```python
from build123d import *

# Parameters (mm, degrees)
F1_DEPTH = 152.4
F2_DEPTH = 25.4
F3_DEPTH = 101.6
F4_DEPTH = 127


with BuildPart() as f1:
    # F0 (on Front) → F1 (new body)
    with BuildSketch(Plane.XZ):
        Polygon((0, 50.8), (0, 0), (304.8, 0), (304.8, 50.8), (165.1, 50.8), (152.4, 50.8), (139.7, 50.8), align=None)
    extrude(amount=F1_DEPTH)

    # F0 (on Front) → F2 (join)
    with BuildSketch(Plane.XZ):
        with BuildLine():
            Line((165.1, 50.8), (304.8, 50.8))
            Line((304.8, 50.8), (233.192970397, 254))
            Line((233.192970397, 254), (228.6, 254))
            ThreePointArc((228.6, 254), (210.5987113259, 204.8131115032), (165.1, 178.8657867546))
            Line((165.1, 178.8657867546), (165.1, 50.8))
        make_face()
        with BuildLine():
            Line((71.607029603, 254), (0, 50.8))
            Line((0, 50.8), (139.7, 50.8))
            Line((139.7, 50.8), (139.7, 178.8657867546))
            ThreePointArc((139.7, 178.8657867546), (94.2012886741, 204.8131115032), (76.2, 254))
            Line((76.2, 254), (71.607029603, 254))
        make_face()
        with BuildLine():
            Line((80.5318662816, 279.3261002888), (71.607029603, 254))
            Line((71.607029603, 254), (76.2, 254))
            ThreePointArc((76.2, 254), (77.2907735716, 266.8469492616), (80.5318662816, 279.3261002888))
        make_face()
        with BuildLine():
            Line((228.6, 254), (233.192970397, 254))
            Line((233.192970397, 254), (224.2681337184, 279.3261002888))
            ThreePointArc((224.2681337184, 279.3261002888), (227.5092264284, 266.8469492616), (228.6, 254))
        make_face()
    extrude(amount=F2_DEPTH)

    # F0 (on Front) → F3 (join)
    with BuildSketch(Plane.XZ):
        with BuildLine():
            Line((152.4, 50.8), (165.1, 50.8))
            Line((165.1, 50.8), (165.1, 178.8657867546))
            ThreePointArc((165.1, 178.8657867546), (158.7723210333, 178.0669141635), (152.4, 177.8))
            Line((152.4, 177.8), (152.4, 50.8))
        make_face()
        with BuildLine():
            Line((139.7, 178.8657867546), (139.7, 50.8))
            Line((139.7, 50.8), (152.4, 50.8))
            Line((152.4, 50.8), (152.4, 177.8))
            ThreePointArc((152.4, 177.8), (146.0276789667, 178.0669141635), (139.7, 178.8657867546))
        make_face()
    extrude(amount=F3_DEPTH)

    # F0 (on Front) → F4 (join)
    with BuildSketch(Plane.XZ):
        with BuildLine():
            ThreePointArc((76.2, 254), (94.2012886741, 204.8131115032), (139.7, 178.8657867546))
            Line((139.7, 178.8657867546), (152.4, 178.8657867546))
            Line((152.4, 178.8657867546), (165.1, 178.8657867546))
            ThreePointArc((165.1, 178.8657867546), (210.5987113259, 204.8131115032), (228.6, 254))
            Line((228.6, 254), (203.2, 254))
            ThreePointArc((203.2, 254), (152.4, 203.2), (101.6, 254))
            Line((101.6, 254), (76.2, 254))
        make_face()
        with BuildLine():
            ThreePointArc((80.5318662816, 279.3261002888), (77.2907735716, 266.8469492616), (76.2, 254))
            Line((76.2, 254), (101.6, 254))
            ThreePointArc((101.6, 254), (152.4, 304.8), (203.2, 254))
            Line((203.2, 254), (228.6, 254))
            ThreePointArc((228.6, 254), (227.5092264284, 266.8469492616), (224.2681337184, 279.3261002888))
            ThreePointArc((224.2681337184, 279.3261002888), (152.4, 330.2), (80.5318662816, 279.3261002888))
        make_face()
        with BuildLine():
            Line((152.4, 178.8657867546), (139.7, 178.8657867546))
            ThreePointArc((139.7, 178.8657867546), (146.0276789667, 178.0669141635), (152.4, 177.8))
            Line((152.4, 177.8), (152.4, 178.8657867546))
        make_face()
        with BuildLine():
            ThreePointArc((152.4, 177.8), (158.7723210333, 178.0669141635), (165.1, 178.8657867546))
            Line((165.1, 178.8657867546), (152.4, 178.8657867546))
            Line((152.4, 178.8657867546), (152.4, 177.8))
        make_face()
    extrude(amount=F4_DEPTH)


solid = f1.part
```
Model file for the job. Use its own axes, mm. A direction names the side the tool comes from. Give positions to 0.01 mm unless a question says otherwise; leave off trailing zeros. Loops run counter-clockwise (first coordinate to the right, second up) from the corner with the lowest first, then second, coordinate; pieces in that order, holes last. Notation, with made-up numbers: M 45.25,62 L 103.25,62 A16 cw 103.25,85 Z; hole C -25.75,28.25 d2. An arc over 180 degrees is marked long. Use one line per item in the form item = value.
Item 1: Which spindle directions (+Z, -Z, +X, -X, +Y, -Y) get a long thin tool onto all of the face, cutting with end or side? Do faces 1 (the flat face through (139.7, -63, 116)), 2 (the flat face through (155, -102, 50.8)), 3 (the flat face through (165.1, -63, 114)). Say none if no direction does.
Filled in:
face_1 = -X, -Y
face_2 = -Y
face_3 = +X, -Y
Item 2: Slice it at C-C on x = 272. List the corners of the cut face in (y, z), and give its area (3 significant figures).
Filled in:
outline = M -152.4,0 L 0,0 L 0,143.88 L -25.4,143.88 L -25.4,50.8 L -152.4,50.8 Z
area = 10,100 mm^2
Item 3: Slice it at A-A on y = -55. List the corners of the cut face in (x, z), and give its area (3 significant figures).
Filled in:
outline = M 0,0 L 304.8,0 L 304.8,50.8 L 165.1,50.8 L 165.1,178.87 A76.2 ccw long 139.7,178.87 L 139.7,50.8 L 0,50.8 Z; hole C 152.4,254 d101.6
area = 28,900 mm^2
Item 4: Drill centre lines: L1, parallel to Z at x = 152.4, y = -94.5; L2, parallel to Z at x = 105.5, y = -86.5; L3, parallel to Z at x = 173, y = -94.5. Where is each one in solid material? Low to high.
Filled in:
L1 = 0 to 203.2, 304.8 to 330.2
L2 = 0 to 50.8, 193.94 to 234.48, 273.52 to 314.06
L3 = 0 to 50.8, 180.64 to 207.56, 300.44 to 327.36
Item 5: Two-plate mould, pull along Z, no slides. Class faces 4 (the flat face through (152, -101.6, 116)), 5 (the flat face through (150, -75, 0)), 6 (the flat face through (150, 0, 131)): released by +Z, released by -Z, zero draft, split by the parting line, or undercut.
Filled in:
face_4 = undercut
face_5 = released by -Z
face_6 = zero draft
Item 6: Slice it at D-D on z = 163.5. List the corners of the cut face in (x, y), and give its area (3 significant figures).
Filled in:
outline = M 39.72,-25.4 L 139.7,-25.4 L 139.7,-101.6 L 165.1,-101.6 L 165.1,-25.4 L 265.08,-25.4 L 265.08,0 L 39.72,0 Z
area = 7,660 mm^2
Item 7: Flat gauge pins, fed straight in: pin 1 Ø12.5 at (x, z) = (147.5, 128.5) entering from -Y; pin 2 Ø1 at (y, z) = (-100.5, 275.5) entering from -X; pin 3 Ø3 at (x, y) = (55, -55.5) entering from +Z. Where does each tip first touch, or does it go through?
Filled in:
pin_1 = -101.6
pin_2 = 79.15
pin_3 = 50.8
Item 8: Slice it at B-B on z = 104. List the corners of the cut face in (x, y).
Filled in:
outline = M 18.75,-25.4 L 139.7,-25.4 L 139.7,-101.6 L 165.1,-101.6 L 165.1,-25.4 L 286.05,-25.4 L 286.05,0 L 18.75,0 Z
